Part model, mm, in its own coordinate system. Face numbers are marked on the shaded views. Round coordinates to 2 decimals unless told otherwise and drop trailing zeros. Loops run counter-clockwise (first coordinate to the right, second up) from the corner with the lowest first, then second, coordinate; pieces in that order, holes last. Notation, with made-up numbers: (76.25, 70.25) - (96.25, 70.25) arc R30 cw to (96.25, 97.25) - close; hole circle Ø5 at (17, -5.75). An arc over 180 degrees is marked (long way). Put each result on its own line as item: value.
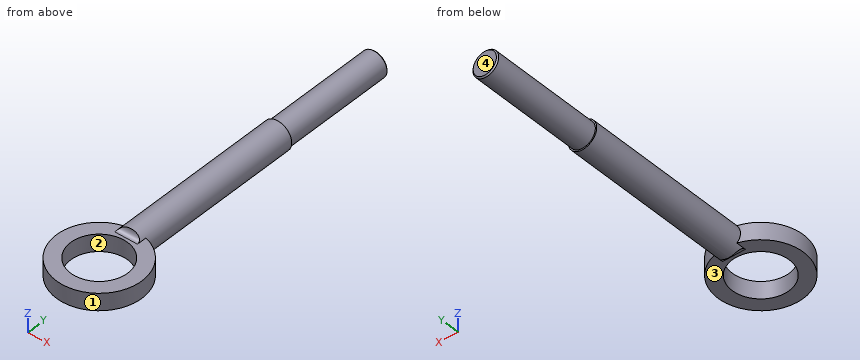
from build123d import *

# Parameters (mm, degrees)
SKETCH1_R                = 2.5
BOSS_EXTRUDE1_DEPTH      = 50
BOSS_EXTRUDE2_DEPTH      = 1.5
BOSS_EXTRUDE2_DEPTH_BACK = 1.5
SKETCH2_R                = 7.5
SKETCH2_R_2              = 5
FILLET1_R                = 1
FILLET2_R                = 1


# Read off the part's stored shape, not the designer's step: M5x0.75 Machine Threads Stud1
with BuildPart() as part:
    # Sketch1 → Boss-Extrude1 (new body)
    with BuildSketch(Plane(origin=(0, 0, 0), x_dir=(1, 0, 0), z_dir=(0, 1, 0))):
        with Locations(Location((0, 0, 0), (0, 0, 270))):
            Circle(SKETCH1_R)
    extrude(amount=BOSS_EXTRUDE1_DEPTH)

    # Sketch2 → Boss-Extrude2 (add, two sides: drawn at the far end of the back side and taken through both)
    with BuildSketch(Plane.XY.offset(-BOSS_EXTRUDE2_DEPTH_BACK)):
        with Locations((0, -6.5)):
            Circle(SKETCH2_R)
        with Locations((0, -6.5)):
            Circle(SKETCH2_R_2, mode=Mode.SUBTRACT)
    extrude(amount=BOSS_EXTRUDE2_DEPTH + BOSS_EXTRUDE2_DEPTH_BACK)

    # Fillet1
    fillet1_edges = [part.edges().sort_by_distance(p)[0] for p in [
        (0, 0, -1.5),
    ]]
    fillet(fillet1_edges, radius=FILLET1_R - 0.0001)  # a hair under: the kernel refuses the full size

    # Fillet2
    fillet2_edges = [part.edges().sort_by_distance(p)[0] for p in [
        (0, 0, 1.5),
    ]]
    fillet(fillet2_edges, radius=FILLET2_R - 0.0001)  # a hair under: the kernel refuses the full size

    # M5x0.75 Machine Threads Stud1 outline → M5x0.75 Machine Threads Stud1 (revolve, cut)
    with BuildSketch(Plane.XY):
        Polygon((2.5, 50), (2.04, 50), (2.2565, 49.7835), (2.2565, 30), (2.5, 30), align=None)
    revolve(axis=Axis((0, 0, 0), (0, 1, 0)), mode=Mode.SUBTRACT)


solid = part.part
1. Probe line 1 along Y through (x, z) = (0, 0.85); line 2 along Y through (x, z) = (-0.75, 0.4); line 3 along X through (y, z) = (36, 1.05). List the from-to ranges inside material, lowest first. Write a range as [from, to].
A:
line 1: y = [-14, -11.5], [-1.5, 50]
line 2: y = [-13.96, -11.44], [-1.56, 50]
line 3: x = [-2, 2]
2. Band-saw the part on A-A (y = -6.5). List the corners of the cut face in (x, z), plus the area to 3 significant figures.
A:
outline: (-7.5, -1.5) - (-5, -1.5) - (-5, 1.5) - (-7.5, 1.5) - close; (5, -1.5) - (7.5, -1.5) - (7.5, 1.5) - (5, 1.5) - close
area: 15.0 mm²
3. Pin check, flat tips, straight feed: P1, Ø7.5, axis at x = -2, y = -3.5, coming from the +Z side; P2, Ø3, axis at x = 4, z = 0, coming from the -Y side; P3, Ø8, axis at x = -3.5, y = 21, coming from the -Z side; P4, Ø1.5, axis at y = -2, z = 1, coming from the +X side. Stop position of each tip, or through.
A:
P1: stops at z = 2.42
P2: stops at y = -13.57
P3: stops at z = -2.5
P4: stops at x = 6.5
4. Two-plate mould, pull along Y, no slides. Class the marked faces 1, 2, 3 and 4: pulls with the +Y half, pulls with the -Y half, needs draft (parallel to the pull), parting line crosses it, or undercut.
A:
face 1: parting line crosses it
face 2: undercut
face 3: needs draft
face 4: pulls with the +Y half
5. Band-saw the part on D-D (y = 8.5). List the corners of the cut face in (x, z), plus the area to 3 significant figures.
A:
outline: circle Ø5 at (0, 0)
area: 19.6 mm²
6. Band-saw the part on C-C (z = 0). List the corners of the cut face in (x, y), plus the area to 3 significant figures.
A:
outline: (-2.5, 0.57) arc R7.5 ccw (long way) to (2.5, 0.57) - (2.5, 30) - (2.26, 30) - (2.26, 49.78) - (2.04, 50) - (-2.04, 50) - (-2.26, 49.78) - (-2.26, 30) - (-2.5, 30) - close; hole circle Ø10 at (0, -6.5)
area: 334 mm²
7. Band-saw the part on B-B (x = 4.25). List the corners of the cut face in (y, z), plus the area to 3 significant figures.
A:
outline: (-12.68, -1.5) - (-9.13, -1.5) - (-9.13, 1.5) - (-12.68, 1.5) - close; (-3.87, -1.5) - (-0.32, -1.5) - (-0.32, 1.5) - (-3.87, 1.5) - close
area: 21.3 mm²
